```python
from build123d import *

# Parameters (mm, degrees)
SKETCH_1_W          = 106
SKETCH_1_H          = 40
EXTRUDE_1_DEPTH     = 3
CUT_EXTRUDE_1_REACH = 58.727
SKETCH_2_R          = 4.25
SKETCH_2_R_2        = 2.75
CUT_EXTRUDE_2_REACH = 58.727
SKETCH_3_R          = 1.6
CUT_EXTRUDE_3_REACH = 58.727


with BuildPart() as part:
    # 草图1 → 凸台-拉伸1 (new body)
    with BuildSketch(Plane(origin=(0, 0, 0), x_dir=(1, 0, 0), z_dir=(0, 1, 0))):
        Rectangle(SKETCH_1_W, SKETCH_1_H)
    extrude(amount=EXTRUDE_1_DEPTH)

    # 草图2 → 切除-拉伸1 (cut, up to next)
    with BuildSketch(Plane(origin=(0, 3, 0), x_dir=(1, 0, 0), z_dir=(0, 1, 0)), mode=Mode.PRIVATE) as cut_extrude_1_sk1:
        with Locations(Location((-31.5, 0, 0), (0, 0, 270))):
            Circle(SKETCH_2_R)
    cut_extrude_1_tool1 = extrude(cut_extrude_1_sk1.sketch, amount=-CUT_EXTRUDE_1_REACH, mode=Mode.PRIVATE) & part.part
    # 草图2 → 切除-拉伸1 (cut, up to next)
    with BuildSketch(Plane(origin=(0, 3, 0), x_dir=(1, 0, 0), z_dir=(0, 1, 0)), mode=Mode.PRIVATE) as cut_extrude_1_sk2:
        with Locations(Location((31.5, 0, 0), (0, 0, 270))):
            Circle(SKETCH_2_R)
    cut_extrude_1_tool2 = extrude(cut_extrude_1_sk2.sketch, amount=-CUT_EXTRUDE_1_REACH, mode=Mode.PRIVATE) & part.part
    # 草图2 → 切除-拉伸1 (cut, up to next)
    with BuildSketch(Plane(origin=(0, 3, 0), x_dir=(1, 0, 0), z_dir=(0, 1, 0)), mode=Mode.PRIVATE) as cut_extrude_1_sk3:
        with Locations(Location((-47.5, 0, 0), (0, 0, 270))):
            Circle(SKETCH_2_R_2)
    cut_extrude_1_tool3 = extrude(cut_extrude_1_sk3.sketch, amount=-CUT_EXTRUDE_1_REACH, mode=Mode.PRIVATE) & part.part
    # 草图2 → 切除-拉伸1 (cut, up to next)
    with BuildSketch(Plane(origin=(0, 3, 0), x_dir=(1, 0, 0), z_dir=(0, 1, 0)), mode=Mode.PRIVATE) as cut_extrude_1_sk4:
        with Locations(Location((-15.5, 0, 0), (0, 0, 270))):
            Circle(SKETCH_2_R_2)
    cut_extrude_1_tool4 = extrude(cut_extrude_1_sk4.sketch, amount=-CUT_EXTRUDE_1_REACH, mode=Mode.PRIVATE) & part.part
    # 草图2 → 切除-拉伸1 (cut, up to next)
    with BuildSketch(Plane(origin=(0, 3, 0), x_dir=(1, 0, 0), z_dir=(0, 1, 0)), mode=Mode.PRIVATE) as cut_extrude_1_sk5:
        with Locations(Location((15.5, 0, 0), (0, 0, 270))):
            Circle(SKETCH_2_R_2)
    cut_extrude_1_tool5 = extrude(cut_extrude_1_sk5.sketch, amount=-CUT_EXTRUDE_1_REACH, mode=Mode.PRIVATE) & part.part
    # 草图2 → 切除-拉伸1 (cut, up to next)
    with BuildSketch(Plane(origin=(0, 3, 0), x_dir=(1, 0, 0), z_dir=(0, 1, 0)), mode=Mode.PRIVATE) as cut_extrude_1_sk6:
        with Locations(Location((47.5, 0, 0), (0, 0, 270))):
            Circle(SKETCH_2_R_2)
    cut_extrude_1_tool6 = extrude(cut_extrude_1_sk6.sketch, amount=-CUT_EXTRUDE_1_REACH, mode=Mode.PRIVATE) & part.part
    add(cut_extrude_1_tool1.solids().sort_by_distance((-31.5, 3, 0))[0], mode=Mode.SUBTRACT)
    add(cut_extrude_1_tool2.solids().sort_by_distance((31.5, 3, 0))[0], mode=Mode.SUBTRACT)
    add(cut_extrude_1_tool3.solids().sort_by_distance((-47.5, 3, 0))[0], mode=Mode.SUBTRACT)
    add(cut_extrude_1_tool4.solids().sort_by_distance((-15.5, 3, 0))[0], mode=Mode.SUBTRACT)
    add(cut_extrude_1_tool5.solids().sort_by_distance((15.5, 3, 0))[0], mode=Mode.SUBTRACT)
    add(cut_extrude_1_tool6.solids().sort_by_distance((47.5, 3, 0))[0], mode=Mode.SUBTRACT)

    # 草图3 → 切除-拉伸2 (cut, up to next)
    with BuildSketch(Plane(origin=(0, 3, 0), x_dir=(1, 0, 0), z_dir=(0, 1, 0)), mode=Mode.PRIVATE) as cut_extrude_2_sk1:
        with Locations(Location((-15.5, -15.5, 0), (0, 0, 270))):
            Circle(SKETCH_3_R)
    cut_extrude_2_tool1 = extrude(cut_extrude_2_sk1.sketch, amount=-CUT_EXTRUDE_2_REACH, mode=Mode.PRIVATE) & part.part
    # 草图3 → 切除-拉伸2 (cut, up to next)
    with BuildSketch(Plane(origin=(0, 3, 0), x_dir=(1, 0, 0), z_dir=(0, 1, 0)), mode=Mode.PRIVATE) as cut_extrude_2_sk2:
        with Locations(Location((-15.5, 15.5, 0), (0, 0, 270))):
            Circle(SKETCH_3_R)
    cut_extrude_2_tool2 = extrude(cut_extrude_2_sk2.sketch, amount=-CUT_EXTRUDE_2_REACH, mode=Mode.PRIVATE) & part.part
    # 草图3 → 切除-拉伸2 (cut, up to next)
    with BuildSketch(Plane(origin=(0, 3, 0), x_dir=(1, 0, 0), z_dir=(0, 1, 0)), mode=Mode.PRIVATE) as cut_extrude_2_sk3:
        with Locations(Location((15.5, 15.5, 0), (0, 0, 270))):
            Circle(SKETCH_3_R)
    cut_extrude_2_tool3 = extrude(cut_extrude_2_sk3.sketch, amount=-CUT_EXTRUDE_2_REACH, mode=Mode.PRIVATE) & part.part
    # 草图3 → 切除-拉伸2 (cut, up to next)
    with BuildSketch(Plane(origin=(0, 3, 0), x_dir=(1, 0, 0), z_dir=(0, 1, 0)), mode=Mode.PRIVATE) as cut_extrude_2_sk4:
        with Locations(Location((15.5, -15.5, 0), (0, 0, 270))):
            Circle(SKETCH_3_R)
    cut_extrude_2_tool4 = extrude(cut_extrude_2_sk4.sketch, amount=-CUT_EXTRUDE_2_REACH, mode=Mode.PRIVATE) & part.part
    add(cut_extrude_2_tool1.solids().sort_by_distance((-15.5, 3, 15.5))[0], mode=Mode.SUBTRACT)
    add(cut_extrude_2_tool2.solids().sort_by_distance((-15.5, 3, -15.5))[0], mode=Mode.SUBTRACT)
    add(cut_extrude_2_tool3.solids().sort_by_distance((15.5, 3, -15.5))[0], mode=Mode.SUBTRACT)
    add(cut_extrude_2_tool4.solids().sort_by_distance((15.5, 3, 15.5))[0], mode=Mode.SUBTRACT)

    # 草图4 → 切除-拉伸3 (cut, up to next)
    with BuildSketch(Plane(origin=(0, 3, 0), x_dir=(1, 0, 0), z_dir=(0, 1, 0)), mode=Mode.PRIVATE) as cut_extrude_3_sk1:
        Polygon((-6, 5.5), (-4.5, 5.5), (-4.5, -1.5), (-9.5, -1.5), (-9.5, 5.5), (-8, 5.5), (-8, 11.5), (-6, 11.5), align=None)
    cut_extrude_3_tool1 = extrude(cut_extrude_3_sk1.sketch, amount=-CUT_EXTRUDE_3_REACH, mode=Mode.PRIVATE) & part.part
    # 草图4 → 切除-拉伸3 (cut, up to next)
    with BuildSketch(Plane(origin=(0, 3, 0), x_dir=(1, 0, 0), z_dir=(0, 1, 0)), mode=Mode.PRIVATE) as cut_extrude_3_sk2:
        Polygon((8, 11.5), (8, 5.5), (9.5, 5.5), (9.5, -1.5), (4.5, -1.5), (4.5, 5.5), (6, 5.5), (6, 11.5), align=None)
    cut_extrude_3_tool2 = extrude(cut_extrude_3_sk2.sketch, amount=-CUT_EXTRUDE_3_REACH, mode=Mode.PRIVATE) & part.part
    add(cut_extrude_3_tool1.solids().sort_by_distance((-7, 3, -3.659574))[0], mode=Mode.SUBTRACT)
    add(cut_extrude_3_tool2.solids().sort_by_distance((7, 3, -3.659574))[0], mode=Mode.SUBTRACT)


solid = part.part
```
The listing builds one solid part. Answer for the finished solid, in the listing's coordinates (mm). A direction names the side the tool comes from. Give positions to 0.01 mm unless a question says otherwise; leave off trailing zeros. Order: outer loops, then holes, each group sorted by start corner. A loop starts at its lowest first (then second) coordinate and runs counter-clockwise, first axis right, second up. Notation, with made-up numbers: M -31,-2.75 L 28,-2.75 A16 cw 28,18.25 Z; hole C 39.5,-2.5 d2. An arc over 180 degrees is marked long. Put each result on its own line as item: value. Start each with the question number.
Item 1: Find the intervals of material crossed by line 1 along X through (y, z) = (2.5, -15.5); line 2 along X through (y, z) = (1.95, -8); line 3 along Z through (x, y) = (5, 1.4), in increasing order.
Item 2: The part is cut by section A-A, the plane z = 15.5. Determine the outline of the cut face in (x, y), and give its area (3 significant figures).
Item 3: For a pull along X with two mould halves and no side action, classify faces 1 (the face through (53, 1, 0)), 2 (the face through (-1, 1, 20)), 3 (the face through (-12.773, 1.521, -0.358)), 4 (the face through (-7, 2, 1.5)) as +X half, -X half, draft (parallel to the pull), parting line (faces both ways), or undercut.
Item 4: The part is cut by section C-C, the plane x = -15.5. Determine the outline of the cut face in (y, z), and give its area (3 significant figures).
Item 5: Which of the six approach directions +Z, -Z, +X, -X, +Y, -Y give full straight-line access (tool end or side, diameter ignored) to faces 5 (the face through (-53, 1, 0)), 6 (the face through (9.5, 2, -2))?
Item 6: The part is cut by section B-B, the plane x = -47.5. Determine the outline of the cut face in (y, z).
Item 7: The part is cut by section D-D, the plane y = 1.5. State how many separate pieces and enclosed holes the cut face has, and give its area (3 significant figures).
Answer key:
1. line 1: x = -53 to -17.1, -13.9 to 13.9, 17.1 to 53
1. line 2: x = -53 to -8, -6 to 6, 8 to 53
1. line 3: z = -20 to -5.5, 1.5 to 20
2. outline: M -53,0 L -17.1,0 L -17.1,3 L -53,3 Z; M -13.9,0 L 13.9,0 L 13.9,3 L -13.9,3 Z; M 17.1,0 L 53,0 L 53,3 L 17.1,3 Z
2. area: 299 mm²
3. face 1: +X half
3. face 2: draft
3. face 3: undercut
3. face 4: undercut
4. outline: M 0,-20 L 3,-20 L 3,-17.1 L 0,-17.1 Z; M 0,-13.9 L 3,-13.9 L 3,-2.75 L 0,-2.75 Z; M 0,2.75 L 3,2.75 L 3,13.9 L 0,13.9 Z; M 0,17.1 L 3,17.1 L 3,20 L 0,20 Z
4. area: 84.3 mm²
5. face 5: +Z, -Z, -X, +Y, -Y
5. face 6: +Y, -Y
6. outline: M 0,-20 L 3,-20 L 3,-2.75 L 0,-2.75 Z; M 0,2.75 L 3,2.75 L 3,20 L 0,20 Z
7. separate pieces: 1
7. enclosed holes: 12
7. area: 3,910 mm²
